from build123d import *

# Parameters (mm, degrees)
SKETCH1_W           = 50
SKETCH1_H           = 40
BOSS_EXTRUDE1_DEPTH = 10
SKETCH5_W           = 6
SKETCH5_H           = 5
BOSS_EXTRUDE3_DEPTH = 10
SKETCH6_R           = 2
CUT_EXTRUDE1_DEPTH  = 20
SKETCH8_W           = 10
SKETCH8_H           = 40
CUT_EXTRUDE2_DEPTH  = 25
SKETCH9_W           = 10
SKETCH9_H           = 6
SKETCH9_R           = 1.930897171
BOSS_EXTRUDE4_DEPTH = 5
SKETCH10_W          = 10
SKETCH10_H          = 5
CUT_EXTRUDE3_DEPTH  = 15
SKETCH11_W          = 5
SKETCH11_H          = 5
BOSS_EXTRUDE5_DEPTH = 10
SKETCH12_R          = 1.5
CUT_EXTRUDE4_DEPTH  = 10
SKETCH13_W          = 6
SKETCH13_H          = 5
CUT_EXTRUDE5_DEPTH  = 10
SKETCH15_W          = 5
SKETCH15_H          = 5
BOSS_EXTRUDE7_DEPTH = 10
SKETCH18_W          = 5
SKETCH18_H          = 5
CUT_EXTRUDE7_DEPTH  = 10
SKETCH19_R          = 1.5
CUT_EXTRUDE8_DEPTH  = 43
CUT_EXTRUDE9_DEPTH  = 20
SKETCH21_W          = 31
SKETCH21_H          = 31
CUT_EXTRUDE10_DEPTH = 30
SKETCH22_W          = 20
SKETCH22_H          = 4.999197144
CUT_EXTRUDE11_DEPTH = 2


with BuildPart() as part:
    # Sketch1 → Boss-Extrude1 (new body)
    with BuildSketch(Plane(origin=(669.84184187, 0, 0), x_dir=(1, 0, 0), z_dir=(0, 0, 1))):
        with Locations((-671.310344828, 437.637931034)):
            Rectangle(SKETCH1_W, SKETCH1_H)
    boss_extrude1 = extrude(amount=BOSS_EXTRUDE1_DEPTH)

    # Sketch5 → Boss-Extrude3 (add)
    with BuildSketch(Plane(origin=(23.531497042, 0, 0), x_dir=(0, 0, -1), z_dir=(1, 0, 0))):
        with Locations((-5, 442.637931034)):
            Rectangle(SKETCH5_W, SKETCH5_H)
        with Locations((-5, 432.637931034)):
            Rectangle(SKETCH5_W, SKETCH5_H)
    extrude(amount=BOSS_EXTRUDE3_DEPTH)

    # Sketch6 → Cut-Extrude1 (cut)
    with BuildSketch(Plane(origin=(669.84184187, 445.137931034, 0), x_dir=(1, 0, 0), z_dir=(0, 1, 0))):
        with Locations(Location((-641.310344828, -5, 0), (0, 0, 180))):
            Circle(SKETCH6_R)
    extrude(amount=-CUT_EXTRUDE1_DEPTH, mode=Mode.SUBTRACT)

    # Sketch8 → Cut-Extrude2 (cut)
    with BuildSketch(Plane.ZY.offset(26.468502958)):
        with Locations((5, 437.637931034)):
            Rectangle(SKETCH8_W, SKETCH8_H)
    extrude(amount=-CUT_EXTRUDE2_DEPTH, mode=Mode.SUBTRACT)

    # Sketch9 → Boss-Extrude4 (add)
    with BuildSketch(Plane(origin=(0, 435.137931034, 0), x_dir=(1, 0, 0), z_dir=(0, 1, 0))):
        with Locations((28.531497042, -5)):
            Rectangle(SKETCH9_W, SKETCH9_H)
        with Locations(Location((28.531497042, -5, 0), (0, 0, 180))):
            Circle(SKETCH9_R, mode=Mode.SUBTRACT)
    extrude(amount=BOSS_EXTRUDE4_DEPTH)

    # Sketch10 → Cut-Extrude3 (cut)
    with BuildSketch(Plane.XY.offset(8)):
        with Locations((28.531497042, 432.637931034)):
            Rectangle(SKETCH10_W, SKETCH10_H)
        with Locations((28.531497042, 442.637931034)):
            Rectangle(SKETCH10_W, SKETCH10_H)
    extrude(amount=-CUT_EXTRUDE3_DEPTH, mode=Mode.SUBTRACT)

    # Mirror1: Boss-Extrude1 across plane
    add(boss_extrude1.mirror(Plane(origin=(-1.468502958, 0, 0), x_dir=(0, 0, 1), z_dir=(1, 0, 0))))

    # Sketch11 → Boss-Extrude5 (add)
    with BuildSketch(Plane(origin=(0, 457.637931034, 0), x_dir=(1, 0, 0), z_dir=(0, 1, 0))):
        with Locations((-1.468502958, -5)):
            Rectangle(SKETCH11_W, SKETCH11_H)
    extrude(amount=BOSS_EXTRUDE5_DEPTH)

    # Sketch12 → Cut-Extrude4 (cut)
    with BuildSketch(Plane(origin=(1.031497042, 0, 0), x_dir=(0, 0, -1), z_dir=(1, 0, 0))):
        with Locations((-5, 462.637931034)):
            Circle(SKETCH12_R)
    extrude(amount=-CUT_EXTRUDE4_DEPTH, mode=Mode.SUBTRACT)

    # Sketch13 → Cut-Extrude5 (cut)
    with BuildSketch(Plane(origin=(33.531497042, 0, 0), x_dir=(0, 0, -1), z_dir=(1, 0, 0))):
        with Locations((-5, 437.637931034)):
            Rectangle(SKETCH13_W, SKETCH13_H)
    extrude(amount=-CUT_EXTRUDE5_DEPTH, mode=Mode.SUBTRACT)

    # Sketch15 → Boss-Extrude7 (add)
    with BuildSketch(Plane(origin=(0, 457.637931034, 0), x_dir=(1, 0, 0), z_dir=(0, 1, 0))):
        with Locations((-6.468502958, -5)):
            Rectangle(SKETCH15_W, SKETCH15_H)
        with Locations((3.531497042, -5)):
            Rectangle(SKETCH15_W, SKETCH15_H)
    extrude(amount=BOSS_EXTRUDE7_DEPTH)

    # Sketch18 → Cut-Extrude7 (cut)
    with BuildSketch(Plane(origin=(0, 467.637931034, 0), x_dir=(1, 0, 0), z_dir=(0, 1, 0))):
        with Locations((-1.468502958, -5)):
            Rectangle(SKETCH18_W, SKETCH18_H)
    extrude(amount=-CUT_EXTRUDE7_DEPTH, mode=Mode.SUBTRACT)

    # Sketch19 → Cut-Extrude8 (cut)
    with BuildSketch(Plane.ZY.offset(8.968502958)):
        with Locations((5, 462.637931034)):
            Circle(SKETCH19_R)
    extrude(amount=-CUT_EXTRUDE8_DEPTH, mode=Mode.SUBTRACT)

    # Sketch20 → Cut-Extrude9 (cut)
    with BuildSketch(Plane(origin=(6.031497042, 0, 0), x_dir=(0, 0, -1), z_dir=(1, 0, 0))):
        with BuildLine():
            Line((-7.5, 467.637931034), (-7.5, 462.637931034))
            ThreePointArc((-7.5, 462.637931034), (-5, 465.137931034), (-2.5, 462.637931034))
            Line((-2.5, 462.637931034), (-2.5, 467.637931034))
            Line((-2.5, 467.637931034), (-7.5, 467.637931034))
        make_face()
    extrude(amount=-CUT_EXTRUDE9_DEPTH, mode=Mode.SUBTRACT)

    # Sketch21 → Cut-Extrude10 (cut)
    with BuildSketch(Plane.XY.offset(10)):
        with Locations((-1.468502958, 437.637931034)):
            Rectangle(SKETCH21_W, SKETCH21_H)
    extrude(amount=-CUT_EXTRUDE10_DEPTH, mode=Mode.SUBTRACT)

    # Sketch22 → Cut-Extrude11 (cut)
    with BuildSketch(Plane(origin=(0, 0, 0), x_dir=(-1, 0, 0), z_dir=(0, 0, -1))):
        with Locations((1.468502958, 455.138332462)):
            Rectangle(SKETCH22_W, SKETCH22_H)
    extrude(amount=-CUT_EXTRUDE11_DEPTH, mode=Mode.SUBTRACT)


solid = part.part
Source: CAD feature listing. Evaluate the final solid. Frame: model axes, mm. A direction names the side the tool comes from. Coordinates: 2 decimals unless noted, no trailing zeros. Write each loop counter-clockwise with the first axis right and the second up, starting at its lowest first coordinate (ties: lowest second). Pieces come first, ordered by that corner, then holes. Notation, with made-up numbers: M -3.75,1.5 L 55.25,1.5 A3 ccw 55.25,6.5 Z; hole C 2,84 d11. An arc over 180 degrees is marked long. Use a Markdown table: item, result.
1) Section B-B, the plane z = 5. Output: boundary loops of the cut face in (x, y), then the cut area to 3 significant figures.
Conclusion:
| item | result |
|---|---|
| outline | M -26.47,417.64 L 23.53,417.64 L 23.53,457.64 L 6.03,457.64 L 6.03,461.14 L 1.03,461.14 L 1.03,457.64 L -3.97,457.64 L -3.97,461.14 L -8.97,461.14 L -8.97,457.64 L -26.47,457.64 Z; M -8.97,464.14 L -3.97,464.14 L -3.97,465.14 L -8.97,465.14 Z; M 1.03,464.14 L 6.03,464.14 L 6.03,465.14 L 1.03,465.14 Z; hole M -16.97,422.14 L 14.03,422.14 L 14.03,453.14 L -16.97,453.14 Z |
| area | 1,080 mm^2 |
2) Ray query, L1, parallel to Y at x = 4.7, z = 5; L2, parallel to X at y = 425.5, z = 5.5; L3, parallel to Y at x = -5, z = 8. Return the intervals inside material, ascending.
Conclusion:
| item | result |
|---|---|
| L1 | y = 417.64 to 422.14, 453.14 to 461.14, 464.14 to 465.14 |
| L2 | x = -26.47 to -16.97, 14.03 to 23.53 |
| L3 | y = 417.64 to 422.14, 453.14 to 457.64 |
3) First-contact query: pin 1 Ø4 at (y, z) = (462.64, 5) entering from -X; pin 2 Ø3 at (x, z) = (9, 4.5) entering from +Y; pin 3 Ø5.5 at (x, y) = (2.5, 460.5) entering from +Z. Flat tips, straight axial feed; report the tip coordinate or a pass-through.
Conclusion:
| item | result |
|---|---|
| pin 1 | stops at x = -8.97 |
| pin 2 | stops at y = 457.64 |
| pin 3 | stops at z = 7.5 |
4) Mould query, pull axis Z, two halves, no side actions, for faces 4 (the cylindrical face through (-6.504, 461.307, 5.692)), 5 (the flat face through (-7, 460, 2.5)), 6 (the cylindrical face through (-6.434, 465.137, 5.055)). Classes: pulls with the +Z half, pulls with the -Z half, needs draft (parallel to the pull), parting line crosses it, or undercut.
Conclusion:
| item | result |
|---|---|
| face 4 | undercut |
| face 5 | pulls with the -Z half |
| face 6 | parting line crosses it |
5) Section C-C, the plane y = 447. Output: boundary loops of the cut face in (x, z).
Conclusion:
| item | result |
|---|---|
| outline | M -26.47,0 L -16.97,0 L -16.97,10 L -26.47,10 Z; M 14.03,0 L 23.53,0 L 23.53,10 L 14.03,10 Z |
6) Section D-D, the plane z = 9.25. Output: boundary loops of the cut face in (x, y), then the cut area to 3 significant figures.
Conclusion:
| item | result |
|---|---|
| outline | M -26.47,417.64 L 23.53,417.64 L 23.53,457.64 L -26.47,457.64 Z; hole M -16.97,422.14 L 14.03,422.14 L 14.03,453.14 L -16.97,453.14 Z |
| area | 1,040 mm^2 |
7) Section A-A, the plane x = 3. Output: boundary loops of the cut face in (y, z), then the cut area to 3 significant figures.
Conclusion:
| item | result |
|---|---|
| outline | M 417.64,0 L 422.14,0 L 422.14,10 L 417.64,10 Z; M 453.14,2 L 457.64,2 L 457.64,2.5 L 462.64,2.5 A2.5 ccw 462.64,7.5 L 457.64,7.5 L 457.64,10 L 453.14,10 Z; hole C 462.64,5 d3 |
| area | 109 mm^2 |
8) Reachability of faces 1 (the flat face through (3, 460, 7.5)), 2 (the flat face through (-1, 455, 2)), 3 (the flat face through (14.031, 437, 5)) from +Z, -Z, +X, -X, +Y, -Y: full face, straight path, thin tool, end or side. Return the list, or none.
Conclusion:
| item | result |
|---|---|
| face 1 | +Z, +X, -X, +Y |
| face 2 | -Z, +Y |
| face 3 | +Z, -Z |
